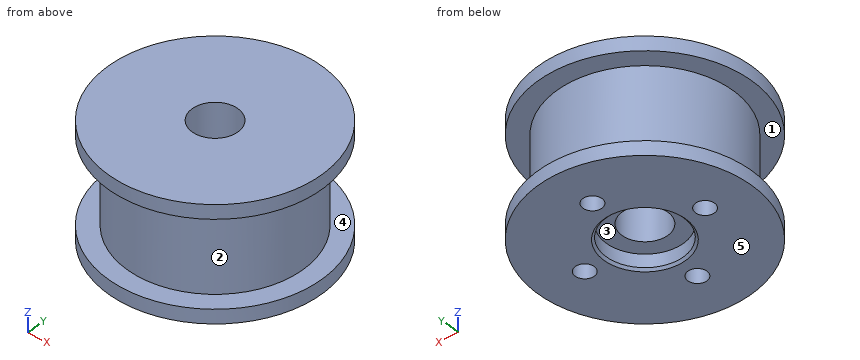
```python
from build123d import *

# Parameters (mm, degrees)
CIRPATTERN2_COUNT       = 4
CHAMFER1_SIZE           = 0.3
CHAMFER2_SIZE           = 0.15
SKETCH6_R               = 5.05
CUT_EXTRUDE1_DEPTH      = 2
CHAMFER3_SIZE           = 0.3
SKETCH7_R               = 8
CUT_EXTRUDE2_DEPTH      = 6
CUT_EXTRUDE3_DEPTH      = 26.39125592
CUT_EXTRUDE3_DEPTH_BACK = 26.39125592
SKETCH10_R              = 22.04861813
SKETCH10_R_2            = 14


with BuildPart() as part:
    # Cut-Revolve1: read off the stored shape, not the designer's step
    # Cut-Revolve1 outline → Cut-Revolve1 (revolve)
    with BuildSketch(Plane.XZ):
        Polygon((11.525, 2.46), (15, 2.46), (16, 2.765730681), (15.628687935, 3.980237722), (14.810197228, 3.73), (8, 3.73), (8, 9.73), (3, 9.73), (3, -11.27), (14.810197228, -11.27), (15.628687935, -11.520237722), (16, -10.305730681), (15, -10), (11.525, -10), align=None)
    revolve(axis=Axis((0, 0, 0), (0, 0, 1)))

    # Sketch4 → M3 Tapped Hole2 (revolve, cut)
    with BuildSketch(Plane(origin=(0, -8, -11.27), x_dir=(0, 1, 0), z_dir=(1, 0, 0))):
        Polygon((0, 0), (0, 9.251075774), (1.25, 8.5), (1.25, 0), align=None)
    m3_tapped_hole2 = revolve(axis=Axis((0, -8, -17.62), (0, 0, 1)), mode=Mode.SUBTRACT)

    # CirPattern2: M3 Tapped Hole2 ×4 about axis
    cirpattern2_axis = Axis((0, 0, 0), (0, 0, 1))
    for i in range(1, CIRPATTERN2_COUNT):
        add(m3_tapped_hole2.rotate(cirpattern2_axis, i * 360 / CIRPATTERN2_COUNT), mode=Mode.SUBTRACT)

    # Chamfer1
    chamfer1_edges = [part.edges().sort_by_distance(p)[0] for p in [
        (-8, 0, 9.73),
    ]]
    chamfer(chamfer1_edges, length=CHAMFER1_SIZE)

    # Chamfer2
    chamfer2_edges = [part.edges().sort_by_distance(p)[0] for p in [
        (-3, 0, 9.73),
    ]]
    chamfer(chamfer2_edges, length=CHAMFER2_SIZE)

    # Sketch6 → Cut-Extrude1 (cut)
    with BuildSketch(Plane(origin=(0, 0, -11.27), x_dir=(-1, 0, 0), z_dir=(0, 0, -1))):
        Circle(SKETCH6_R)
    extrude(amount=-CUT_EXTRUDE1_DEPTH, mode=Mode.SUBTRACT)

    # Chamfer3
    chamfer3_edges = [part.edges().sort_by_distance(p)[0] for p in [
        (5.05, 0, -11.27),
    ]]
    chamfer(chamfer3_edges, length=CHAMFER3_SIZE)

    # Sketch7 → Cut-Extrude2 (cut)
    with BuildSketch(Plane.XY.offset(9.73)):
        Circle(SKETCH7_R)
    extrude(amount=-CUT_EXTRUDE2_DEPTH, mode=Mode.SUBTRACT)

    # Sketch9 → Revolve1 (revolve)
    with BuildSketch(Plane(origin=(0, 0, 0), x_dir=(1, 0, 0), z_dir=(0, 1, 0))):
        Polygon((-16, 10.305730681), (-14.85, 9.42), (-11.525, 9.42), (-11.525, 10.305730681), align=None)
        Polygon((-16, -2.765730681), (-14.85, -1.88), (-11.525, -1.88), (-11.525, -2.765730681), align=None)
    revolve(axis=Axis((0, 0, -10.305730681), (0, 0, 1)))

    # Sketch10 → Cut-Extrude3 (cut, two sides: drawn at the far end of the back side and taken through both)
    with BuildSketch(Plane.XY.offset(-CUT_EXTRUDE3_DEPTH_BACK)):
        Circle(SKETCH10_R)
        with Locations(Location((0, 0, 0), (0, 0, 180))):
            Circle(SKETCH10_R_2, mode=Mode.SUBTRACT)
    extrude(amount=CUT_EXTRUDE3_DEPTH + CUT_EXTRUDE3_DEPTH_BACK, mode=Mode.SUBTRACT)


solid = part.part
```
The listing builds one solid part. Answer for the finished solid, in the listing's coordinates (mm). Face numbers are marked on the shaded views. A direction names the side the tool comes from. Give positions to 0.01 mm unless a question says otherwise; leave off trailing zeros. Order: outer loops, then holes, each group sorted by start corner. A loop starts at its lowest first (then second) coordinate and runs counter-clockwise, first axis right, second up. Notation, with made-up numbers: (1, -21.5) - (11, -21.5) arc R25 ccw to (11, 4.5) - close; hole circle Ø6 at (71, 68). An arc over 180 degrees is marked (long way). Use one line per item in the form item = value. Start each with the question number.
(1) For the marked faces 4 and 5, determine the directions among +Z, -Z, +X, -X, +Y, -Y from which every point of the face is accessible in a straight line to the end or side of a thin tool.
(2) Flat-ended cylindrical pins translate along their axes: pin 1 Ø3 at (y, z) = (-7.5, -1) entering from +X; pin 2 Ø5 at (y, z) = (-5, -1) entering from -X; pin 3 Ø4 at (x, y) = (8, 0) entering from -Z; pin 4 Ø3 at (x, z) = (-4.5, -3.5) entering from +Y. Find the tip coordinate at first contact, or state that the pin passes through.
(3) The mould has two halves that part along Y. Classify the marked faces 1, 2 and 3: released by +Y, released by -Y, zero draft, split by the parting line, or undercut.
(4) A cutting plane is placed at C-C, the plane z = -0.5. Write down the section's boundary in (x, y) (3 decimals), then the cut area to 3 significant figures.
(5) A cutting plane is placed at A-A, the plane z = -6.5. Write down the section's boundary in (x, y) (3 decimals), then the cut area to 3 significant figures.
(6) A cutting plane is placed at B-B, the plane x = -11. Write down the section's boundary in (y, z).
(7) Consider line 1 (X direction, y = -1, z = -7.5); line 2 (Y direction, x = 1, z = 2); line 3 (Z direction, x = 12.75, y = 3.75). Determine where each line is inside the solid, lowest interval first. Write a range as from..to.
Ans:
q1.face_4 = none
q1.face_5 = -Z, +X, -X, +Y, -Y
q2.pin_1 = 9.84
q2.pin_2 = -11.25
q2.pin_3 = -11.27
q2.pin_4 = 11.13
q3.face_1 = zero draft
q3.face_2 = split by the parting line
q3.face_3 = undercut
q4.outline = circle Ø23.05 at (0, 0); hole circle Ø6 at (0, 0)
q4.area = 389 mm^2
q5.outline = circle Ø23.05 at (0, 0); hole circle Ø2.5 at (-8, 0); hole circle Ø6 at (0, 0); hole circle Ø2.5 at (0, -8); hole circle Ø2.5 at (0, 8); hole circle Ø2.5 at (8, 0)
q5.area = 369 mm^2
q6.outline = (-8.66, -11.27) - (8.66, -11.27) - (8.66, -9.42) - (3.44, -9.42) - (3.44, 1.88) - (8.66, 1.88) - (8.66, 3.73) - (-8.66, 3.73) - (-8.66, 1.88) - (-3.44, 1.88) - (-3.44, -9.42) - (-8.66, -9.42) - close
q7.line_1 = -11.48..-8.75, -7.25..-2.83, 2.83..7.25, 8.75..11.48
q7.line_2 = -13.96..-2.83, 2.83..13.96
q7.line_3 = -11.27..-9.42, 1.88..3.73
